Verification items for the finished model (mm, model axes). A direction names the side the tool comes from. Round coordinates to 2 decimals unless told otherwise and drop trailing zeros. Order: outer loops, then holes, each group sorted by start corner. A loop starts at its lowest first (then second) coordinate and runs counter-clockwise, first axis right, second up.
```python
from build123d import *

# Parameters (mm, degrees)
BOSS_EXTRUDE1_DEPTH     = 1.1
SKETCH2_R               = 3.4
BOSS_EXTRUDE2_DEPTH     = 3.4
CUT_EXTRUDE1_DEPTH      = 11.119487388
CUT_EXTRUDE1_DEPTH_BACK = 11.119487388
CUT_EXTRUDE2_DEPTH      = 2
BOSS_EXTRUDE3_DEPTH     = 0.15
BOSS_EXTRUDE4_DEPTH     = 3.4
CUT_EXTRUDE3_START      = -3.4
CUT_EXTRUDE3_DEPTH      = 1.55
SKETCH10_W              = 0.475
SKETCH10_H              = 1.905
CUT_EXTRUDE4_DEPTH      = 10.486518065


with BuildPart() as part:
    # Sketch1 → Boss-Extrude1 (new body)
    with BuildSketch(Plane.XY):
        Polygon((-1.84, 8.4), (-3.405, 6.65), (-3.405, 1.55), (-2.8, 1), (2.8, 1), (3.405, 1.55), (3.405, 6.65), (1.84, 8.4), align=None)
    extrude(amount=BOSS_EXTRUDE1_DEPTH)

    # Sketch2 → Boss-Extrude2 (add)
    with BuildSketch(Plane.XY.offset(1.1)):
        with Locations(Location((0, 5, 0), (0, 0, 180))):
            Circle(SKETCH2_R)
    extrude(amount=BOSS_EXTRUDE2_DEPTH)

    # Sketch3 → Cut-Extrude1 (cut, two sides: drawn at the far end of the back side and taken through both)
    with BuildSketch(Plane(origin=(0, 0, 0), x_dir=(0, 0, -1), z_dir=(1, 0, 0)).offset(-CUT_EXTRUDE1_DEPTH_BACK)):
        Polygon((-3.15, 8.4), (-3.15, 7.4), (-4.5, 6.8), (-4.5, 8.4), align=None)
    extrude(amount=CUT_EXTRUDE1_DEPTH + CUT_EXTRUDE1_DEPTH_BACK, mode=Mode.SUBTRACT)

    # Sketch5 → Cut-Revolve1 (revolve, cut)
    with BuildSketch(Plane(origin=(0, 5, 0), x_dir=(-1, 0, 0), z_dir=(0, 1, 0)), mode=Mode.PRIVATE) as cut_revolve1_sk:
        Polygon((0, 4.5), (-1.9, 4.5), (-0.425, 3.37), (0, 3.37), align=None)
    revolve(cut_revolve1_sk.sketch.rotate(Axis((0, 5, 3.37), (0, 0, 1)), 148.034281249), axis=Axis((0, 5, 3.37), (0, 0, 1)), mode=Mode.SUBTRACT)

    # Sketch6 → Cut-Extrude2 (cut)
    with BuildSketch(Plane.XY.offset(4.5)):
        with BuildLine():
            Line((0.425, 5.425), (1.851857176, 5.425))
            ThreePointArc((1.851857176, 5.425), (1.9, 5), (1.851857176, 4.575))
            Line((1.851857176, 4.575), (0.425, 4.575))
            Line((0.425, 4.575), (0.425, 3.148142824))
            ThreePointArc((0.425, 3.148142824), (0, 3.1), (-0.425, 3.148142824))
            Line((-0.425, 3.148142824), (-0.425, 4.575))
            Line((-0.425, 4.575), (-1.851857176, 4.575))
            ThreePointArc((-1.851857176, 4.575), (-1.9, 5), (-1.851857176, 5.425))
            Line((-1.851857176, 5.425), (-0.425, 5.425))
            Line((-0.425, 5.425), (-0.425, 6.851857176))
            ThreePointArc((-0.425, 6.851857176), (0, 6.9), (0.425, 6.851857176))
            Line((0.425, 6.851857176), (0.425, 5.425))
        make_face()
    extrude(amount=-CUT_EXTRUDE2_DEPTH, mode=Mode.SUBTRACT)

    # Sketch7 → Boss-Extrude3 (add, symmetric)
    with BuildSketch(Plane.XY):
        with BuildLine():
            Line((-0.425, 0.21), (-0.425, -1.905))
            Line((-0.425, -1.905), (0.425, -1.905))
            Line((0.425, -1.905), (0.425, 0.21))
            Line((0.425, 0.21), (0.875, 0.21))
            Line((0.875, 0.21), (0.875, 1))
            ThreePointArc((0.875, 1), (0, 1.875), (-0.875, 1))
            Line((-0.875, 1), (-0.875, 0.21))
            Line((-0.875, 0.21), (-0.425, 0.21))
        make_face()
    extrude(amount=BOSS_EXTRUDE3_DEPTH, both=True)

    # Sketch8 → Boss-Extrude4 (add, symmetric)
    with BuildSketch(Plane(origin=(0, 0, 0), x_dir=(0, 0, -1), z_dir=(1, 0, 0))):
        with BuildLine():
            Line((0, 1.85), (-1.9, 1.85))
            ThreePointArc((-1.9, 1.85), (-2.430330086, 1.630330086), (-2.65, 1.1))
            Line((-2.65, 1.1), (-2.65, -1.905))
            Line((-2.65, -1.905), (-2.35, -1.905))
            Line((-2.35, -1.905), (-2.35, 1.1))
            ThreePointArc((-2.35, 1.1), (-2.218198052, 1.418198052), (-1.9, 1.55))
            Line((-1.9, 1.55), (0, 1.55))
            Line((0, 1.55), (0, 1.85))
        make_face()
    extrude(amount=BOSS_EXTRUDE4_DEPTH, both=True)

    # Sketch9 → Cut-Extrude3 (cut)
    with BuildSketch(Plane.XY.offset(4.5).offset(CUT_EXTRUDE3_START)):
        with BuildLine():
            Line((-2.075, -1.905), (-2.075, 2.306605302))
            ThreePointArc((-2.075, 2.306605302), (0, 1.6), (2.075, 2.306605302))
            Line((2.075, 2.306605302), (2.075, -1.905))
            Line((2.075, -1.905), (-2.075, -1.905))
        make_face()
    extrude(amount=CUT_EXTRUDE3_DEPTH, mode=Mode.SUBTRACT)

    # Sketch10 → Cut-Extrude4 (cut, through all)
    with BuildSketch(Plane.XY.offset(2.65)):
        with Locations((-3.1625, -0.9525)):
            Rectangle(SKETCH10_W, SKETCH10_H)
        with Locations((3.1625, -0.9525)):
            Rectangle(SKETCH10_W, SKETCH10_H)
    extrude(amount=-CUT_EXTRUDE4_DEPTH, mode=Mode.SUBTRACT)


solid = part.part
```
1) Scan lines: probe 1 along Z at (x, y) = (-1, 2.25); probe 2 along Z at (x, y) = (-1.5, 5.25); probe 3 along X at (y, z) = (6.5, 4.15) (3 decimals). Record each from-to range of solid material in increasing order.
2) Sectioned sample at D-D on z = 2.05. Record the cut outline in (x, y) (3 decimals).
3) Sectioned sample at C-C on y = 5. Record the cut outline in (x, z) (3 decimals), then the cut area to 3 significant figures.
4) Go/stop test with flat-tipped pins: pin 1 Ø3 at (x, y) = (-1.5, 5.5) entering from -Z; pin 2 Ø1.7 at (y, z) = (0.5, 2) entering from +X; pin 3 Ø1.5 at (x, z) = (-1.5, 1.5) entering from -Y. Record where each tip stops, or that it passes through.
5) Tool access check on faces 5 (the flat face through (0, 0, 0.15)), 6 (the flat face through (2.633, 7.513, 0.542)), 7 (the conical face through (0.972, 4.012, 4.106)). Record the directions out of +Z, -Z, +X, -X, +Y, -Y that give a thin tool (end or side, any length) a straight path to the whole face; none if there is none.
6) Sectioned sample at B-B on z = 3.85. Record the cut outline in (x, y) (3 decimals), then the cut area to 3 significant figures.
7) Sectioned sample at A-A on z = 0.7. Record the cut outline in (x, y) (3 decimals), then the cut area to 3 significant figures.
8) Draft check along X on faces 1 (the flat face through (0.425, 4, 3)), 2 (the flat face through (-2.6, -0.4, 2.65)), 3 (the flat face through (-3.405, 4.1, 0.5)), 4 (the flat face through (-1, 4.575, 3)). Enter one of: released by +X, released by -X, zero draft, split by the parting line, or undercut.
Returned:
1. probe 1: z = 0 to 4.5
1. probe 2: z = 0 to 2.5
1. probe 3: x = -3.051 to -0.425, 0.425 to 3.051
2. outline: (-3.4, 1.524) - (-2.075, 1.524) - (-2.075, 1.835) - (-3.4, 1.835) - close; circle Ø6.8 at (0, 5); (2.075, 1.524) - (3.4, 1.524) - (3.4, 1.835) - (2.075, 1.835) - close
3. outline: (-3.405, 0) - (3.405, 0) - (3.405, 1.1) - (3.4, 1.1) - (3.4, 4.5) - (1.9, 4.5) - (1.9, 2.5) - (-1.9, 2.5) - (-1.9, 4.5) - (-3.4, 4.5) - (-3.4, 1.1) - (-3.405, 1.1) - close
3. area: 23.0 mm2
4. pin 1: stops at z = 0
4. pin 2: stops at x = 3.4
4. pin 3: stops at y = 1
5. face 5: +Z, +X, -X, -Y
5. face 6: +Z, -Z, +X, +Y
5. face 7: +Z
6. outline: (-2.683, 7.089) arc R3.4 ccw (long way) to (2.683, 7.089) - close; hole (-1.852, 4.575) - (-0.962, 4.575) arc R1.052 ccw to (-0.425, 4.038) - (-0.425, 3.148) arc R1.9 ccw to (0.425, 3.148) - (0.425, 4.038) arc R1.052 ccw to (0.962, 4.575) - (1.852, 4.575) arc R1.9 ccw to (1.852, 5.425) - (0.962, 5.425) arc R1.052 ccw to (0.425, 5.962) - (0.425, 6.852) arc R1.9 ccw to (-0.425, 6.852) - (-0.425, 5.962) arc R1.052 ccw to (-0.962, 5.425) - (-1.852, 5.425) arc R1.9 ccw to start
6. area: 25.0 mm2
7. outline: (-3.405, 1.55) - (-2.8, 1) - (2.8, 1) - (3.405, 1.55) - (3.405, 6.65) - (1.84, 8.4) - (-1.84, 8.4) - (-3.405, 6.65) - close
7. area: 47.3 mm2
8. face 1: undercut
8. face 2: zero draft
8. face 3: released by -X
8. face 4: undercut
